Autodesk Inventor part; units mm, degrees
ref_plane "YZ Plane" through (0, 0, 0) normal (1, 0, 0) x (0, 1, 0)
ref_plane "XZ Plane" through (0, 0, 0) normal (0, 1, 0) x (-1, 0, 0)
ref_plane "XY Plane" through (0, 0, 0) normal (0, 0, 1) x (1, 0, 0)
sketch "Sketch1" plane through (0, 0, 0) normal (0, 0, 1) x (1, 0, 0)
  line L0 (-32.2735, -28.2023) -> (32.2735, -28.2023)
  line L1 (32.2735, -28.2023) -> (282.2736, 404.8104)
  line L2 (282.2736, 404.8104) -> (250.0001, 460.7098)
  line L3 (250.0001, 460.7098) -> (-249.9999, 460.71)
  line L4 (-249.9999, 460.71) -> (-282.2735, 404.8106)
  line L5 (-282.2735, 404.8106) -> (-32.2735, -28.2023)
  line L6 (0, -28.2023) -> (0, 279.1061)
  line L7 (-266.1368, 432.7601) -> (0, 279.1059)
  line L8 (266.1368, 432.7601) -> (0, 279.1061)
  line L9 (0, 279.1061) -> (0.0001, 460.7099)
  line L10 (0, 279.1061) -> (-157.2735, 188.3042)
  line L11 (0, 279.1059) -> (157.2736, 188.3041)
  point P0 (0, 0)
extrude "Extrusion1" add sketch "Sketch1" along normal blind 18 contours L5 L4 L7 L10 | L7 L4 L3 L9
sketch "Sketch2" plane through (0, 0, 18) normal (0, 0, 1) x (1, 0, 0)
  line L0 (0, 279.1059) -> (0.0001, 460.7099)
  line L1 (0.0001, 460.7099) -> (-249.9999, 460.71)
  line L2 (-249.9999, 460.71) -> (-282.2735, 404.8106)
  line L3 (-282.2735, 404.8106) -> (-157.2735, 188.3042)
  line L4 (-157.2735, 188.3042) -> (0, 279.106)
  line L5 (0, 279.1059) -> (0, 279.106)
  line L6 (-261.5469, 440.71) -> (0.0001, 440.7099)
  line L7 (-139.953, 198.3042) -> (-270.7265, 424.8106)
  point P0 (0, 0)
  dimension "d2" = 20
extrude "Extrusion2" cut sketch "Sketch2" against normal blind 10 contours L4 L7 L2 L6 L0
sketch "Sketch3" plane through (0, 0, 18) normal (0, 0, 1) x (1, 0, 0)
  circle A0 centre (-189.9999, 450.71) radius 2.5
  circle A1 centre (-49.9999, 450.7099) radius 2.5
  circle A2 centre (-243.6132, 357.849) radius 2.5
  circle A3 centre (-173.6132, 236.6055) radius 2.5
  line L0 (0.0001, 460.7099) -> (-249.9999, 460.71)
  line L1 (0.0001, 440.7099) -> (0.0001, 460.7099)
  line L2 (-282.2735, 404.8106) -> (-157.2735, 188.3042)
  line L3 (-157.2735, 188.3042) -> (-139.953, 198.3042)
  point P0 (0, 0)
  dimension "d5" = 5
  dimension "d6" = 5
  dimension "d7" = 5
  dimension "d8" = 5
  dimension "d9" = 10
  dimension "d10" = 10
  dimension "d11" = 50
  dimension "d12" = 190
  dimension "d13" = 10
  dimension "d14" = 10
  dimension "d15" = 50
  dimension "d16" = 190
extrude "Extrusion3" cut sketch "Sketch3" against normal through all
equation "\"d10\" = d9"
equation "\"d13\" = d9"
equation "\"d14\" = d9"
equation "\"d15\" = d11"
equation "\"d16\" = d12"
properties part number "bottom half"
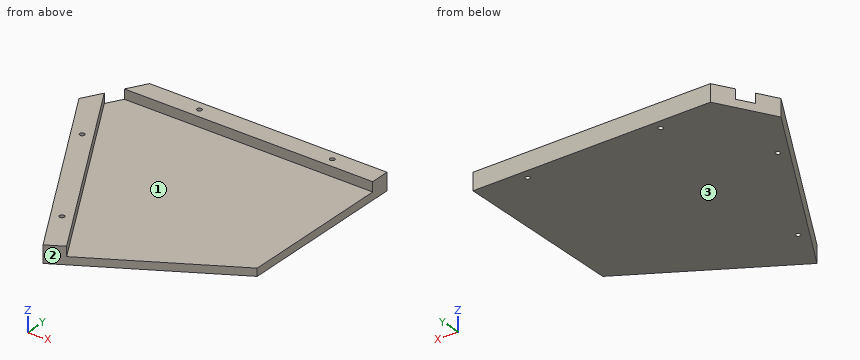
For this review, take the finished solid that the model builds, in its own axes (mm). Face numbers are marked on the shaded views. Give positions to 0.01 mm unless a question says otherwise; leave off trailing zeros. Write each loop counter-clockwise with the first axis right and the second up, starting at its lowest first coordinate (ties: lowest second). Pieces come first, ordered by that corner, then holes.
Item 1: The part is to be moulded in two halves that separate along Y. For the marked faces 1, 2 and 3, say which applies: +Y half, -Y half, draft (parallel to the pull), parting line (faces both ways), or undercut.
Item 2: Wall thickness on probe 1 along X at (y, z) = (450.71, 14.25); probe 2 along Z at (x, y) = (-107.5, 292); probe 3 along Y at (x, z) = (-70, 16.5): over which ranges is each line inside the solid? List them lowest first.
Item 3: Take a section at B-B (y = 283). Give the boundary of the cut face in (x, z), and give its area (3 significant figures).
Item 4: Insertion check: P1, Ø8, axis at x = -169.5, z = 11, coming from the -Y side; P2, Ø5, axis at x = -138.5, z = 7, coming from the -Y side; P3, Ø4, axis at y = 364.5, z = 9.5, coming from the -X side. Each pin has a flat end and moves straight along its axis. Give the tip position at first contact, or say it passes through.
Item 5: Take a section at A-A (z = 13.75). Give the boundary of the cut face in (x, y).
Item 6: Take a section at C-C (x = -77). Give the boundary of the cut face in (y, z).
Established:
1. face 1: undercut
1. face 2: -Y half
1. face 3: draft
2. probe 1: x = -255.77 to -192.5, -187.5 to -52.5, -47.5 to 0
2. probe 2: z = 0 to 8
2. probe 3: y = 440.71 to 460.71
3. outline: (-211.95, 0) - (0, 0) - (0, 8) - (-188.85, 8) - (-188.85, 18) - (-211.95, 18) - close
3. area: 1,930 mm2
4. P1: stops at y = 202.55
4. P2: stops at y = 197.7
4. P3: stops at x = -260.15
5. outline: (-282.27, 404.81) - (-157.27, 188.3) - (-139.95, 198.3) - (-270.73, 424.81) - close; (-261.55, 440.71) - (0, 440.71) - (0, 460.71) - (-250, 460.71) - close; hole circle Ø5 at (-243.61, 357.85); hole circle Ø5 at (-190, 450.71); hole circle Ø5 at (-173.61, 236.61); hole circle Ø5 at (-50, 450.71)
6. outline: (234.65, 0) - (460.71, 0) - (460.71, 18) - (440.71, 18) - (440.71, 8) - (234.65, 8) - close
